Can you work these out from the drawing? Everything is in mm from the part's minimum corner. Give positions to 0.01 mm unless a question says otherwise; leave off trailing zeros. Write each loop counter-clockwise with the first axis right and the second up, starting at its lowest first coordinate (ties: lowest second). Pieces come first, ordered by that corner, then holes. Notation, with made-up numbers: (4, -40) -> (16, -40) arc R13 cw to (16, -35) -> close; hole circle Ø1 at (11, 62). An arc over 180 degrees is marked (long way). Write item = value, one per line. Start each with the question number.
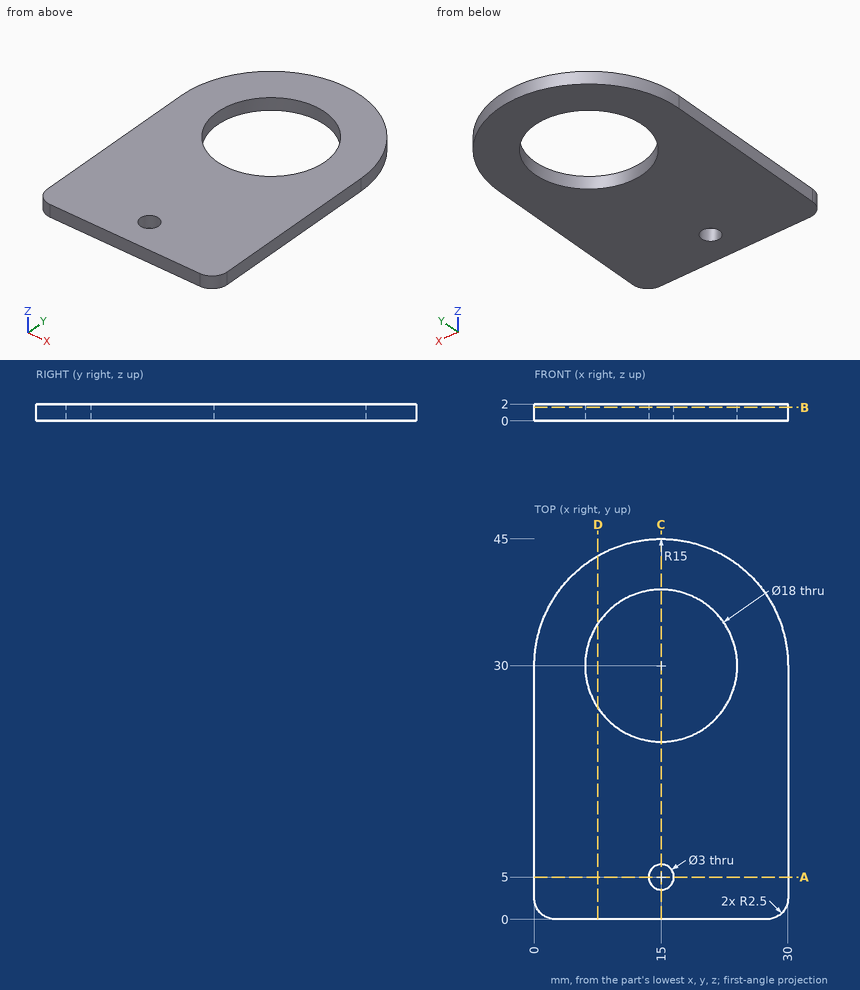
(1) If I drill on line 1 along Y through (x, z) = (15, 1.1); line 2 along Y through (x, z) = (14, 0.65); line 3 along X through (y, z) = (6, 0.7), over which ranges is the centre line in solid material (lowest first)? Write a range as from..to.
(2) I'm going to push a flat-ended pin straight in: pin 1 (1 mm diameter, centred on y = 16.5, z = 1, fed in from -X). Where does the tip first touch, or does it pass through?
(3) Imagine slicing it at A-A (y = 5). Please give me the cut outline in (x, z).
(4) Imagine slicing it at B-B (z = 1.6). Please give me the cut outline in (x, y).
(5) Imagine slicing it at D-D (x = 7.5). Please give me the cut outline in (y, z).
(6) Imagine slicing it at C-C (x = 15). Please give me the cut outline in (y, z).
Answers below:
q1.line_1 = 0..3.5, 6.5..21, 39..45
q1.line_2 = 0..3.88, 6.12..21.06, 38.94..44.97
q1.line_3 = 0..13.88, 16.12..30
q2.pin_1 = 0
q3.outline = (0, 0) -> (13.5, 0) -> (13.5, 2) -> (0, 2) -> close; (16.5, 0) -> (30, 0) -> (30, 2) -> (16.5, 2) -> close
q4.outline = (0, 2.5) arc R2.5 ccw to (2.5, 0) -> (27.5, 0) arc R2.5 ccw to (30, 2.5) -> (30, 30) arc R15 ccw to (0, 30) -> close; hole circle Ø18 at (15, 30); hole circle Ø3 at (15, 5)
q5.outline = (0, 0) -> (25.03, 0) -> (25.03, 2) -> (0, 2) -> close; (34.97, 0) -> (42.99, 0) -> (42.99, 2) -> (34.97, 2) -> close
q6.outline = (0, 0) -> (3.5, 0) -> (3.5, 2) -> (0, 2) -> close; (6.5, 0) -> (21, 0) -> (21, 2) -> (6.5, 2) -> close; (39, 0) -> (45, 0) -> (45, 2) -> (39, 2) -> close
